Input: part model. Units: mm. Frame: model coordinates. A direction names the side the tool comes from. Give positions to 0.01 mm unless a question says otherwise; leave off trailing zeros. Loops run counter-clockwise (first coordinate to the right, second up) from the corner with the lowest first, then second, coordinate; pieces in that order, holes last. Notation, with made-up numbers: M 39.25,35.25 L 98.25,35.25 A24 ccw 98.25,58.25 Z; hole C 48.25,-28.5 d5. An arc over 180 degrees is marked long. Answer as a JSON object with one key per item and string values. Group by question number.
1) Section query A-A on z = 0. Return loops of the section in (x, y).
2) Section query D-D on z = 8. Return loops of the section in (x, y), plus the area to 4 significant figures.
3) First-contact query: P1, Ø4, axis at y = 15, z = -9.5, coming from the -X side; P2, Ø4, axis at x = 1.5, y = 8, coming from the +Z side; P3, Ø8, axis at x = 0.5, y = 30.5, coming from the -Z side; P4, Ø1.5, axis at x = 7, z = 2, coming from the -Y side. Flat tips, straight axial feed; report the tip coordinate or a pass-through.
4) Section query B-B on x = -12.5. Return loops of the section in (y, z).
5) Access query for faces 1 (the flat face through (5.5, 1, -11)), 2 (the flat face through (0, 20, -11)), 3 (the flat face through (0, 28, -13)), 4 (the flat face through (16, 19, -4)). Directions: +Z, -Z, +X, -X, +Y, -Y. A direction counts if a zero-diameter tool reaches every point of the face in a straight line with its end or side. Return the directions, or none.
6) Draft query along X for faces 5 (the flat face through (0, 6, 15)), 6 (the flat face through (21, 1, 0)), 7 (the flat face through (-5.5, 1, -11)), 8 (the flat face through (-21, 1, 0)). Return one class per face: +X half, -X half, draft (parallel to the pull), parting line (faces both ways), or undercut.
7) Section query C-C on y = 38. Return loops of the section in (x, z), plus the area to 4 significant figures.
8) Ray query, L1, parallel to Z at x = 0, y = 2; L2, parallel to X at y = 8, z = -4.5; L3, parallel to Z at x = 1.5, y = 3.5. Return the intervals inside material, ascending.
from build123d import *

# Parameters (mm, degrees)
F0_W      = 32
F0_H      = 30
F1_DEPTH  = 45
F2_T      = -2.5
F4_DEPTH  = 32.001
F5_W      = 42
F5_H      = 40
F6_DEPTH  = 2.5
F7_R      = 1.6
F7_R_2    = 4.25
F7_W      = 8
F7_H      = 4
F8_DEPTH  = 45.001
F9_W      = 15
F9_H      = 25
F10_DEPTH = 3
F11_R     = 5
F12_DEPTH = 2


# Not quite as in the source:
# - a fillet or chamfer that OpenCascade refuses, or shapes differently, is made with other operations: its cross-section is extruded or revolved along the edge and cut away or added


with BuildPart() as f1:
    # F0 (on Front) → F1 (new body)
    with BuildSketch(Plane.XZ):
        Rectangle(F0_W, F0_H)
    extrude(amount=-F1_DEPTH)

    # F2
    f2_openings = [f1.faces().sort_by_distance(p)[0] for p in [
        (0, 45, 0),
    ]]
    offset(amount=F2_T, openings=f2_openings)

    # F3 (on face) → F4 (cut, through all)
    with BuildSketch(Plane.YZ.offset(16)):
        Polygon((45, 15), (10, 15), (45, -10), align=None)
    extrude(amount=-F4_DEPTH, mode=Mode.SUBTRACT)

    # F5 (on face) → F6 (join)
    with BuildSketch(Plane.XZ):
        Rectangle(F5_W, F5_H)
    extrude(amount=-F6_DEPTH)

    # F7 (on face) → F8 (cut, through all)
    with BuildSketch(Plane.XZ):
        with Locations((9.5, 0)):
            Circle(F7_R)
        with Locations((-9.5, 0)):
            Circle(F7_R)
        with Locations((0, -8)):
            Circle(F7_R)
        with Locations((0, 8)):
            Circle(F7_R)
        Circle(F7_R_2)
        with Locations((9.5, -10.5)):
            Rectangle(F7_W, F7_H)
        with Locations((-9.5, -10.5)):
            Rectangle(F7_W, F7_H)
    extrude(amount=-F8_DEPTH, mode=Mode.SUBTRACT)

    # F9 (on face) → F10 (join)
    with BuildSketch(Plane.XY.offset(-12.5)):
        with Locations((0, 32.5)):
            Rectangle(F9_W, F9_H)
    extrude(amount=F10_DEPTH)

    # F11 (on face) → F12 (cut)
    with BuildSketch(Plane(origin=(0, 0, -15), x_dir=(1, 0, 0), z_dir=(0, 0, -1))):
        with Locations((0, -28)):
            Circle(F11_R)
    extrude(amount=-F12_DEPTH, mode=Mode.SUBTRACT)

    # F13: fillet of radius 5 on 1 edges, made by hand

    # F13_s1 → F13_t2 (revolve)
    with BuildSketch(Plane.XZ.offset(-28)):
        with BuildLine():
            ThreePointArc((5, -15), (3.2360679775, -13.527864045), (1, -13))
            Line((1, -13), (5, -13))
            Line((5, -13), (5, -15))
        make_face()
    revolve(axis=Axis((0, 28, -13), (0, 0, -1)))


solid = f1.part
Output:
{
 "1": {"outline": "M -21,0 L -11.1,0 L -11.1,2.5 L -13.5,2.5 L -13.5,31 L -16,31 L -16,2.5 L -21,2.5 Z; M -7.9,0 L -4.25,0 L -4.25,2.5 L -7.9,2.5 Z; M 4.25,0 L 7.9,0 L 7.9,2.5 L 4.25,2.5 Z; M 11.1,0 L 21,0 L 21,2.5 L 16,2.5 L 16,31 L 13.5,31 L 13.5,2.5 L 11.1,2.5 Z"},
 "2": {"outline": "M -21,0 L -1.6,0 L -1.6,2.5 L -13.5,2.5 L -13.5,19.8 L -16,19.8 L -16,2.5 L -21,2.5 Z; M 1.6,0 L 21,0 L 21,2.5 L 16,2.5 L 16,19.8 L 13.5,19.8 L 13.5,2.5 L 1.6,2.5 Z", "area": "183.5 mm^2"},
 "3": {"P1": "stops at x = -16", "P2": "stops at z = 15", "P3": "stops at z = -15", "P4": "stops at y = 0"},
 "4": {"outline": "M 0,-20 L 2.5,-20 L 2.5,-15 L 45,-15 L 45,-12.5 L 0,-12.5 Z; M 0,-8.5 L 2.5,-8.5 L 2.5,12.5 L 13.5,12.5 L 10,15 L 2.5,15 L 2.5,20 L 0,20 Z"},
 "5": {"face 1": "-Y", "face 2": "+Z", "face 3": "-Z", "face 4": "+Z, -Z, +X, +Y"},
 "6": {"face 5": "draft", "face 6": "+X half", "face 7": "undercut", "face 8": "-X half"},
 "7": {"outline": "M -16,-15 L 16,-15 L 16,-5 L 13.5,-5 L 13.5,-12.5 L 7.5,-12.5 L 7.5,-9.5 L -7.5,-9.5 L -7.5,-12.5 L -13.5,-12.5 L -13.5,-5 L -16,-5 Z", "area": "162.5 mm^2"},
 "8": {"L1": "z = -20 to -9.6, -6.4 to -4.25, 4.25 to 6.4, 9.6 to 20", "L2": "x = -16 to -13.5, 13.5 to 16", "L3": "z = -15 to -12.5, 12.5 to 15"}
}
